Could you check a few things on this drawing? It's one solid part, dimensions in mm from its lowest x, y, z. A direction names the side the tool comes from. Round coordinates to 2 decimals unless told otherwise and drop trailing zeros. Loops run counter-clockwise (first coordinate to the right, second up) from the corner with the lowest first, then second, coordinate; pieces in that order, holes last. Notation, with made-up numbers: M 78,-16.5 L 102,-16.5 A17 cw 102,6.5 Z; hole C 69,3 d9. An arc over 180 degrees is marked long. Use a Markdown table: item, result. Add a question column.
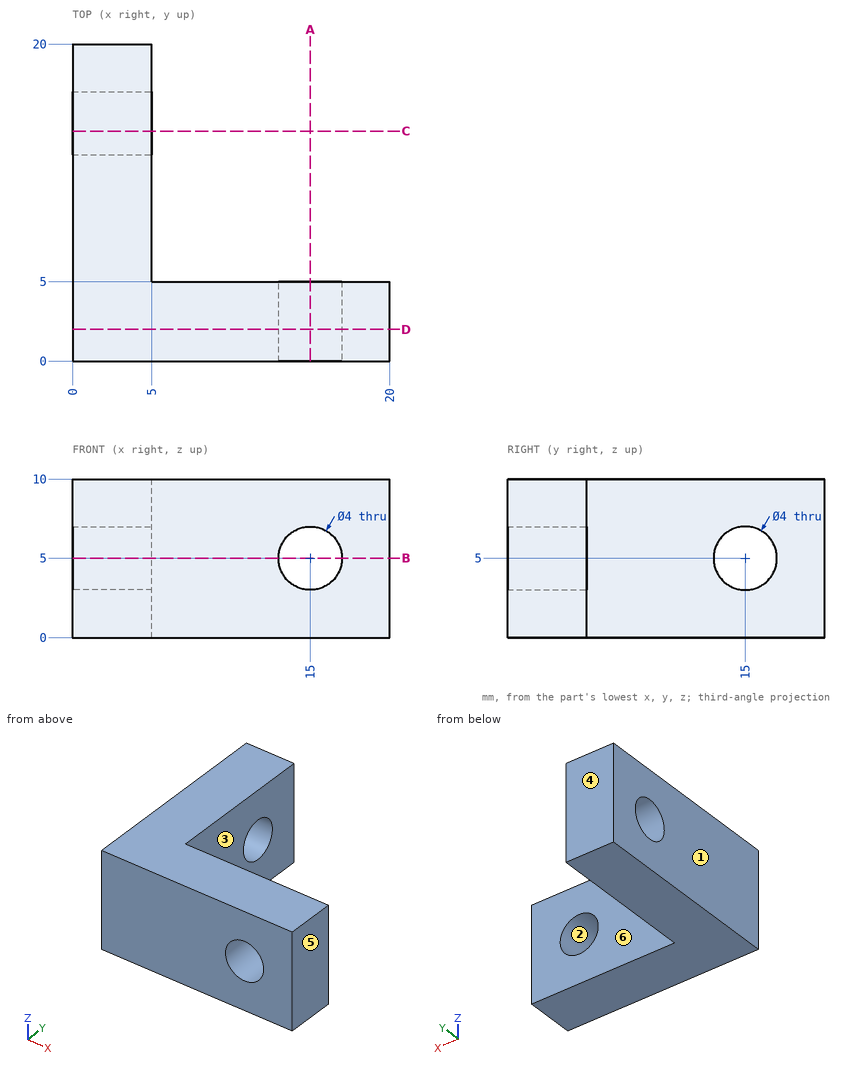
(1) Suppose I cut it at A-A on x = 15. List the corners of the cut face in (y, z) for me.
(2) On a 3-axis mill with a long thin cutter (end or side, diameter ignored), from which of +Z, -Z, +X, -X, +Y, -Y can I reach the whole of each face in a straight line? I mean the marked faces 5 and 6. Say none if no direction works.
(3) Suppose I cut it at D-D on y = 2. List the corners of the cut face in (x, z) for me.
(4) Suppose I cut it at C-C on y = 14.5. List the corners of the cut face in (x, z) for me, and give its area (3 significant figures).
(5) If I drill on probe 1 along X at (y, z) = (1.5, 5); probe 2 along Z at (x, y) = (15, 1.6), over which ranges is the centre line in solid material (lowest first)? Write a range as [from, to].
(6) Thinking about a two-plate mould opening in X: for the marked faces 1, 2, 3 and 4, which applies, released by +X, released by -X, zero draft, split by the parting line, or undercut?
(7) Suppose I cut it at B-B on z = 5. List the corners of the cut face in (x, y) for me, and give its area (3 significant figures).
(8) I'm going to push flat-ended pins straight in: pin 1 (2.5 mm diameter, centred on y = 15, z = 5, fed in from -X); pin 2 (4 mm diameter, centred on x = 9.5, z = 3.5, fed in from +Y); pin 3 (3 mm diameter, centred on y = 11.5, z = 5, fed in from +X). Where does each tip first touch, or does it pass through?
Results below:
| question | item | result |
|---|---|---|
| 1 | outline | M 0,0 L 5,0 L 5,3 L 0,3 Z; M 0,7 L 5,7 L 5,10 L 0,10 Z |
| 2 | face 5 | +Z, -Z, +X, +Y, -Y |
| 2 | face 6 | +Z, -Z, +X, +Y |
| 3 | outline | M 0,0 L 20,0 L 20,10 L 0,10 Z; hole C 15,5 d4 |
| 4 | outline | M 0,0 L 5,0 L 5,3.06 L 0,3.06 Z; M 0,6.94 L 5,6.94 L 5,10 L 0,10 Z |
| 4 | area | 30.6 mm² |
| 5 | probe 1 | x = [0, 13], [17, 20] |
| 5 | probe 2 | z = [0, 3], [7, 10] |
| 6 | face 1 | released by -X |
| 6 | face 2 | undercut |
| 6 | face 3 | released by +X |
| 6 | face 4 | zero draft |
| 7 | outline | M 0,0 L 13,0 L 13,5 L 5,5 L 5,13 L 0,13 Z; M 0,17 L 5,17 L 5,20 L 0,20 Z; M 17,0 L 20,0 L 20,5 L 17,5 Z |
| 7 | area | 135 mm² |
| 8 | pin 1 | passes through |
| 8 | pin 2 | stops at y = 5 |
| 8 | pin 3 | stops at x = 5 |
